Here's how the part is built. I have some questions about the finished solid (model axes, mm). A direction names the side the tool comes from. Round coordinates to 2 decimals unless told otherwise and drop trailing zeros. Loops run counter-clockwise (first coordinate to the right, second up) from the corner with the lowest first, then second, coordinate; pieces in that order, holes last. Notation, with made-up numbers: M 19.5,54.5 L 41.5,54.5 A22 ccw 41.5,61.5 Z; hole C 85.5,12.5 d9. An arc over 180 degrees is marked long. Answer as a JSON object with one key per item and string values.
from build123d import *

# Parameters (mm, degrees)
BENCH_FOOTPRINT_140X120_DEPTH           = 5
BACKBONE_START                          = -20
BACKBONE_PROFILE_W                      = 14
BACKBONE_PROFILE_H                      = 63
BACKBONE_DEPTH                          = 40
REMOVABLE_SERVO_MOUNT_M3_START          = -40
REMOVABLE_SERVO_MOUNT_M3_PROFILE_R      = 1.6
REMOVABLE_SERVO_MOUNT_M3_DEPTH          = 155.560027933
BEARING_BRIDGE_START                    = 39
BEARING_BRIDGE_PROFILE_W                = 53
BEARING_BRIDGE_PROFILE_H                = 40
BEARING_BRIDGE_DEPTH                    = 4
BRIDGE_HORN_CLEARANCE_START             = 38
BRIDGE_HORN_CLEARANCE_PROFILE_R         = 14
BRIDGE_HORN_CLEARANCE_DEPTH             = 77.560027933
DRIVE_COLLAR_CHAMBER_START              = 43
DRIVE_COLLAR_CHAMBER_PROFILE_R          = 18
DRIVE_COLLAR_CHAMBER_PROFILE_R_2        = 14
DRIVE_COLLAR_CHAMBER_DEPTH              = 5
BEARING_TOWER_START                     = 48
BEARING_TOWER_PROFILE_R                 = 18
BEARING_TOWER_PROFILE_R_2               = 11.1
BEARING_TOWER_DEPTH                     = 23
BEARING_SEPARATION_SHOULDER_START       = 55
BEARING_SEPARATION_SHOULDER_PROFILE_R   = 11.1
BEARING_SEPARATION_SHOULDER_PROFILE_R_2 = 9
BEARING_SEPARATION_SHOULDER_DEPTH       = 8
BENCH_CLAMP_HOLES_START                 = -1
BENCH_CLAMP_HOLES_PROFILE_R             = 2.75
BENCH_CLAMP_HOLES_DEPTH                 = 118.365802537
YAW_CROSSBOLT_ACCESS_START              = -40
YAW_CROSSBOLT_ACCESS_PROFILE_R          = 2.5
YAW_CROSSBOLT_ACCESS_DEPTH              = 157.365802537
FILLET2_R                               = 10
BOSS_EXTRUDE1_DEPTH                     = 40
FILLET6_R                               = 1.5
FILLET7_R                               = 10
CHAMFER1_SIZE                           = 10


with BuildPart() as part:
    # Bench_footprint_140x120_profile → Bench_footprint_140x120 (new body)
    with BuildSketch(Plane(origin=(0, 0, 0), x_dir=(1, 0, 0), z_dir=(0, 1, 0))):
        with BuildLine():
            Line((-60, -60), (60, -60))
            ThreePointArc((60, -60), (67.071067812, -57.071067812), (70, -50))
            Line((70, -50), (70, 50))
            ThreePointArc((70, 50), (67.071067812, 57.071067812), (60, 60))
            Line((60, 60), (-60, 60))
            ThreePointArc((-60, 60), (-67.071067812, 57.071067812), (-70, 50))
            Line((-70, 50), (-70, -50))
            ThreePointArc((-70, -50), (-67.071067812, -57.071067812), (-60, -60))
        make_face()
    extrude(amount=BENCH_FOOTPRINT_140X120_DEPTH)

    # Backbone_profile → Backbone (add)
    with BuildSketch(Plane.XY.offset(BACKBONE_START)):
        with Locations((-28, 36.5)):
            Rectangle(BACKBONE_PROFILE_W, BACKBONE_PROFILE_H)
    extrude(amount=BACKBONE_DEPTH)

    # Removable_servo_mount_M3_profile → Removable_servo_mount_M3 (cut, through all)
    with BuildSketch(Plane(origin=(0, 0, 0), x_dir=(0, 0, -1), z_dir=(1, 0, 0)).offset(REMOVABLE_SERVO_MOUNT_M3_START)):
        with Locations(Location((12, 28, 0), (0, 0, 180))):
            Circle(REMOVABLE_SERVO_MOUNT_M3_PROFILE_R)
        with Locations(Location((-12, 28, 0), (0, 0, 180))):
            Circle(REMOVABLE_SERVO_MOUNT_M3_PROFILE_R)
    extrude(amount=REMOVABLE_SERVO_MOUNT_M3_DEPTH, mode=Mode.SUBTRACT)

    # Bearing_bridge_profile → Bearing_bridge (add)
    with BuildSketch(Plane(origin=(0, 0, 0), x_dir=(1, 0, 0), z_dir=(0, 1, 0)).offset(BEARING_BRIDGE_START)):
        with Locations((-8.5, 0)):
            Rectangle(BEARING_BRIDGE_PROFILE_W, BEARING_BRIDGE_PROFILE_H)
    extrude(amount=BEARING_BRIDGE_DEPTH)

    # Bridge_horn_clearance_profile → Bridge_horn_clearance (cut, through all)
    with BuildSketch(Plane(origin=(0, 0, 0), x_dir=(1, 0, 0), z_dir=(0, 1, 0)).offset(BRIDGE_HORN_CLEARANCE_START)):
        with Locations(Location((0, 0, 0), (0, 0, 90))):
            Circle(BRIDGE_HORN_CLEARANCE_PROFILE_R)
    extrude(amount=BRIDGE_HORN_CLEARANCE_DEPTH, mode=Mode.SUBTRACT)

    # Drive_collar_chamber_profile → Drive_collar_chamber (add)
    with BuildSketch(Plane(origin=(0, 0, 0), x_dir=(1, 0, 0), z_dir=(0, 1, 0)).offset(DRIVE_COLLAR_CHAMBER_START)):
        Circle(DRIVE_COLLAR_CHAMBER_PROFILE_R)
        with Locations(Location((0, 0, 0), (0, 0, 90))):
            Circle(DRIVE_COLLAR_CHAMBER_PROFILE_R_2, mode=Mode.SUBTRACT)
    extrude(amount=DRIVE_COLLAR_CHAMBER_DEPTH)

    # Bearing_tower_profile → Bearing_tower (add)
    with BuildSketch(Plane(origin=(0, 0, 0), x_dir=(1, 0, 0), z_dir=(0, 1, 0)).offset(BEARING_TOWER_START)):
        Circle(BEARING_TOWER_PROFILE_R)
        with Locations(Location((0, 0, 0), (0, 0, 270))):
            Circle(BEARING_TOWER_PROFILE_R_2, mode=Mode.SUBTRACT)
    extrude(amount=BEARING_TOWER_DEPTH)

    # Bearing_separation_shoulder_profile → Bearing_separation_shoulder (add)
    with BuildSketch(Plane(origin=(0, 0, 0), x_dir=(1, 0, 0), z_dir=(0, 1, 0)).offset(BEARING_SEPARATION_SHOULDER_START)):
        with Locations(Location((0, 0, 0), (0, 0, 270))):
            Circle(BEARING_SEPARATION_SHOULDER_PROFILE_R)
        with Locations(Location((0, 0, 0), (0, 0, 270))):
            Circle(BEARING_SEPARATION_SHOULDER_PROFILE_R_2, mode=Mode.SUBTRACT)
    extrude(amount=BEARING_SEPARATION_SHOULDER_DEPTH)

    # Bench_clamp_holes_profile → Bench_clamp_holes (cut, through all)
    with BuildSketch(Plane(origin=(0, 0, 0), x_dir=(1, 0, 0), z_dir=(0, 1, 0)).offset(BENCH_CLAMP_HOLES_START)):
        with Locations(Location((-55, -45, 0), (0, 0, 270))):
            Circle(BENCH_CLAMP_HOLES_PROFILE_R)
        with Locations(Location((55, -45, 0), (0, 0, 270))):
            Circle(BENCH_CLAMP_HOLES_PROFILE_R)
        with Locations(Location((-55, 45, 0), (0, 0, 270))):
            Circle(BENCH_CLAMP_HOLES_PROFILE_R)
        with Locations(Location((55, 45, 0), (0, 0, 270))):
            Circle(BENCH_CLAMP_HOLES_PROFILE_R)
    extrude(amount=BENCH_CLAMP_HOLES_DEPTH, mode=Mode.SUBTRACT)

    # Yaw_crossbolt_access_profile → Yaw_crossbolt_access (cut, through all)
    with BuildSketch(Plane(origin=(0, 0, 0), x_dir=(0, 0, -1), z_dir=(1, 0, 0)).offset(YAW_CROSSBOLT_ACCESS_START)):
        with Locations(Location((0, 45.5, 0), (0, 0, 90))):
            Circle(YAW_CROSSBOLT_ACCESS_PROFILE_R)
    extrude(amount=YAW_CROSSBOLT_ACCESS_DEPTH, mode=Mode.SUBTRACT)

    # Fillet2
    fillet2_edges = [part.edges().sort_by_distance(p)[0] for p in [
        (18, 41, -20),
        (18, 41, 20),
    ]]
    fillet(fillet2_edges, radius=FILLET2_R)

    # Sketch1 → Boss-Extrude1 (add)
    with BuildSketch(Plane.XY.offset(20)):
        Polygon((-21, 34), (-16, 39), (-21, 39), align=None)
    extrude(amount=-BOSS_EXTRUDE1_DEPTH)

    # Fillet6
    fillet6_edges = [part.edges().sort_by_distance(p)[0] for p in [
        (-16, 39, 0),
        (-21, 34, 0),
    ]]
    fillet(fillet6_edges, radius=FILLET6_R)

    # Fillet7
    fillet7_edges = [part.edges().sort_by_distance(p)[0] for p in [
        (-28, 5, -20),
        (-35, 5, 0),
        (-21, 5, 0),
        (-28, 5, 20),
    ]]
    fillet(fillet7_edges, radius=FILLET7_R)

    # Chamfer1
    chamfer1_edges = [part.edges().sort_by_distance(p)[0] for p in [
        (-28, 68, -20),
        (-28, 68, 20),
    ]]
    chamfer(chamfer1_edges, length=CHAMFER1_SIZE)


solid = part.part
Item 1: I want a section at A-A on x = -25. List the corners of the cut face in (y, z) for me, plus the area to 3 significant figures.
Solution:
{"outline": "M 0,-60 L 5,-60 L 5,-30 A10 cw 15,-20 L 58,-20 L 68,-10 L 68,10 L 58,20 L 15,20 A10 cw 5,30 L 5,60 L 0,60 Z; hole C 28,-12 d3.2; hole C 28,12 d3.2; hole C 45.5,0 d5", "area": "3,030 mm2"}
Item 2: For faces 5 (the face through (-28, 68, 0)), 6 (the face through (-28, 63, -15)), 7 (the face through (-19, 36, 0)), which set-ups out of +Z, -Z, +X, -X, +Y, -Y let a thin tool reach every point of the face, with its end or its side?
Solution:
{"face 5": "+Z, -Z, -X, +Y", "face 6": "-Z, -X, +Y", "face 7": "+Z, -Z, +X"}
Item 3: If I drill on L1, parallel to X at y = 51.25, z = 0; L2, parallel to X at y = 1.45, z = 45; L3, parallel to Z at x = -15.6, y = 45.5, over which ranges is the centre line in solid material (lowest first)? Write a range as from..to.
Solution:
{"L1": "x = -35..-21, -18..-11.1, 11.1..18", "L2": "x = -70..-57.75, -52.25..52.25, 57.75..70", "L3": "z = -8.98..-2.5, 2.5..8.98"}
Item 4: I want a section at D-D on y = 45.5. List the corners of the cut face in (x, z) for me.
Solution:
{"outline": "M -35,-20 L -21,-20 L -21,-2.5 L -35,-2.5 Z; M -35,2.5 L -21,2.5 L -21,20 L -35,20 Z; M -17.83,-2.5 A18 ccw 17.83,-2.5 L 13.77,-2.5 A14 cw -13.77,-2.5 Z; M -17.83,2.5 L -13.77,2.5 A14 cw 13.77,2.5 L 17.83,2.5 A18 ccw Z"}
Item 5: I want a section at B-B on y = 28. List the corners of the cut face in (x, z) for me, plus the area to 3 significant figures.
Solution:
{"outline": "M -35,-20 L -21,-20 L -21,-13.6 L -35,-13.6 Z; M -35,-10.4 L -21,-10.4 L -21,10.4 L -35,10.4 Z; M -35,13.6 L -21,13.6 L -21,20 L -35,20 Z", "area": "470 mm2"}
Item 6: We'd pull the mould along X, two halves only. Please class faces 1 (the face through (-35, 41, 0)), 2 (the face through (-4.21, 48, -10.44)), 3 (the face through (-19, 43, -2)), 4 (the face through (-28, 7, -24)): +X half, -X half, draft (parallel to the pull), parting line (faces both ways), or undercut.
Solution:
{"face 1": "-X half", "face 2": "undercut", "face 3": "undercut", "face 4": "draft"}
Item 7: I want a section at C-C on x = 55. List the corners of the cut face in (y, z) for me, plus the area to 3 significant figures.
Solution:
{"outline": "M 0,-60 L 5,-60 L 5,-47.75 L 0,-47.75 Z; M 0,-42.25 L 5,-42.25 L 5,42.25 L 0,42.25 Z; M 0,47.75 L 5,47.75 L 5,60 L 0,60 Z", "area": "545 mm2"}
Item 8: For P1, Ø20, axis at y = 23, z = -8, coming from the +X side; P2, Ø4, axis at y = 28, z = 12, coming from the +X side; P3, Ø5, axis at x = -55, z = -45, coming from the +Y side; P4, Ø3, axis at y = 36.5, z = -2, coming from the -X side, each with a flat end and sliding along its axis, tell me the tip position at first contact or that it passes through.
Solution:
{"P1": "stops at x = -20.8", "P2": "stops at x = -21", "P3": "passes through", "P4": "stops at x = -35"}
